Could you check a few things on this drawing? It's one solid part, dimensions in mm from its lowest x, y, z. A direction names the side the tool comes from. Give positions to 0.01 mm unless a question says otherwise; leave off trailing zeros. Order: outer loops, then holes, each group sorted by start corner. A loop starts at its lowest first (then second) coordinate and runs counter-clockwise, first axis right, second up.
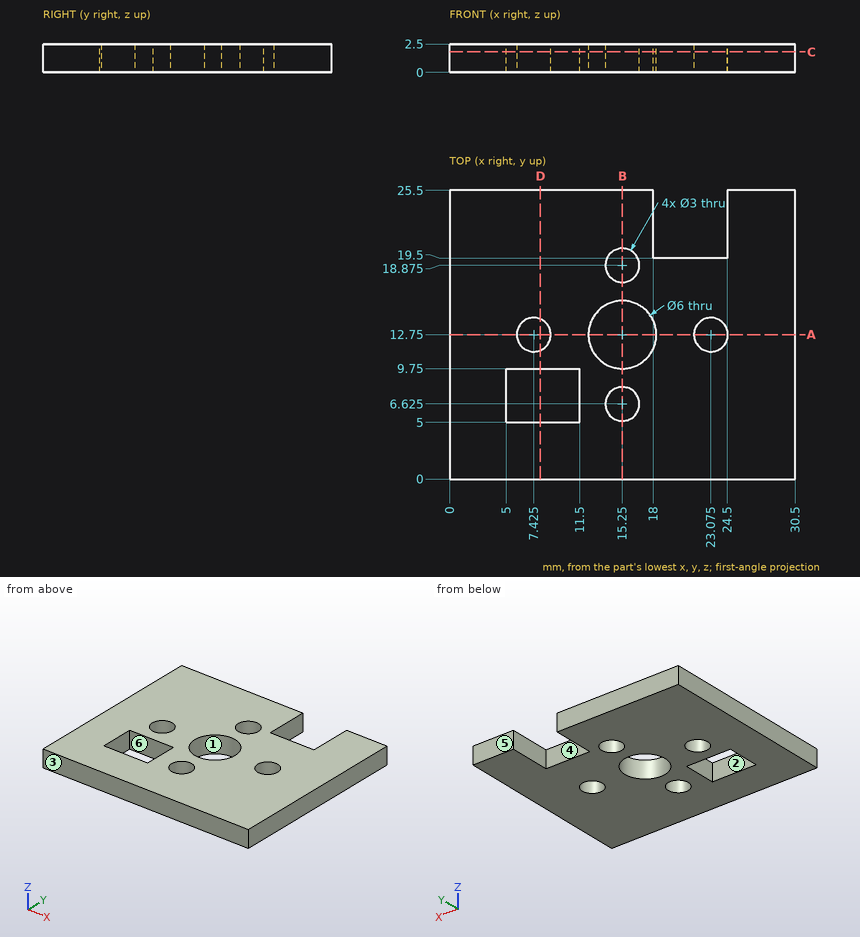
Q1. If we section it at B-B on x = 15.25: List the corners of the cut face in (y, z) for me (3 decimals).
Filled sheet:
outline: (0, 0) - (5.125, 0) - (5.125, 2.5) - (0, 2.5) - close; (8.125, 0) - (9.75, 0) - (9.75, 2.5) - (8.125, 2.5) - close; (15.75, 0) - (17.375, 0) - (17.375, 2.5) - (15.75, 2.5) - close; (20.375, 0) - (25.5, 0) - (25.5, 2.5) - (20.375, 2.5) - close
Q2. If we section it at A-A on y = 12.75: List the corners of the cut face in (x, z) for me (3 decimals).
Filled sheet:
outline: (0, 0) - (5.925, 0) - (5.925, 2.5) - (0, 2.5) - close; (8.925, 0) - (12.25, 0) - (12.25, 2.5) - (8.925, 2.5) - close; (18.25, 0) - (21.575, 0) - (21.575, 2.5) - (18.25, 2.5) - close; (24.575, 0) - (30.5, 0) - (30.5, 2.5) - (24.575, 2.5) - close
Q3. I'm going to push a flat-ended pin straight in: P1, Ø1.2, axis at x = 21, z = 1.5, coming from the +Y side. Where does the tip first touch, or does it pass through?
Filled sheet:
P1: stops at y = 19.5
Q4. For the marked faces 5 and 6, which set-ups out of +Z, -Z, +X, -X, +Y, -Y let a thin tool reach every point of the face, with its end or its side?
Filled sheet:
face 5: +Z, -Z, +X, -X, +Y
face 6: +Z, -Z
Q5. If we section it at D-D on x = 8: List the corners of the cut face in (y, z) for me.
Filled sheet:
outline: (0, 0) - (5, 0) - (5, 2.5) - (0, 2.5) - close; (9.75, 0) - (11.36, 0) - (11.36, 2.5) - (9.75, 2.5) - close; (14.14, 0) - (25.5, 0) - (25.5, 2.5) - (14.14, 2.5) - close
Q6. If we section it at C-C on z = 1.8: List the corners of the cut face in (x, y) for me (3 decimals), plus the area to 3 significant figures.
Filled sheet:
outline: (0, 0) - (30.5, 0) - (30.5, 25.5) - (24.5, 25.5) - (24.5, 19.5) - (18, 19.5) - (18, 25.5) - (0, 25.5) - close; hole (5, 5) - (11.5, 5) - (11.5, 9.75) - (5, 9.75) - close; hole circle Ø3 at (7.425, 12.75); hole circle Ø6 at (15.25, 12.75); hole circle Ø3 at (15.25, 6.625); hole circle Ø3 at (15.25, 18.875); hole circle Ø3 at (23.075, 12.75)
area: 651 mm2
Q7. I need wall thicknesses on L1, parallel to Y at x = 15.25, z = 0.7 (3 decimals); L2, parallel to X at y = 21.5, z = 1.05; L3, parallel to Y at x = 10, z = 2.25. Which ranges of each line are inside material? Lowest first, please.
Filled sheet:
L1: y = 0 to 5.125, 8.125 to 9.75, 15.75 to 17.375, 20.375 to 25.5
L2: x = 0 to 18, 24.5 to 30.5
L3: y = 0 to 5, 9.75 to 25.5
Q8. Thinking about a two-plate mould opening in Y: for the marked faces 1, 2, 3 and 4, which applies, released by +Y, released by -Y, zero draft, split by the parting line, or undercut?
Filled sheet:
face 1: undercut
face 2: undercut
face 3: released by -Y
face 4: released by +Y
